Can you work these out from the model? Positions are in its coordinate system, mm. A direction names the side the tool comes from. Round coordinates to 2 decimals unless told otherwise and drop trailing zeros. Write each loop counter-clockwise with the first axis right and the second up, starting at its lowest first coordinate (ties: lowest second). Pieces come first, ordered by that corner, then holes. Notation, with made-up numbers: M -2,3 L 8,3 A4 ccw 8,10 Z; hole C 51,-4.75 d2. An arc over 180 degrees is marked long. Use one line per item in the form item = value. Start each with the question number.
```python
from build123d import *

# Parameters (mm, degrees)
BOX044_W         = 24
BOX044_H         = 42
BOX044_DEPTH     = 13
SKETCH022_R      = 5
SKETCH022_R_2    = 4.5
SKETCH022_R_3    = 1.25
EXTRUDE022_DEPTH = 3
BOX039_W         = 3
BOX039_H         = 2
BOX039_DEPTH     = 2


with BuildPart() as cube005:
    # Box044 → Box044 (new body)
    with BuildSketch(Plane(origin=(-12, -2, 12), x_dir=(1, 0, 0), z_dir=(0, 0, 1))):
        with Locations((12, 21)):
            Rectangle(BOX044_W, BOX044_H)
    extrude(amount=BOX044_DEPTH)


with BuildPart() as back_cover:
    # Sketch022 → Extrude022 (new body)
    with BuildSketch(Plane.XZ):
        with BuildLine():
            ThreePointArc((10, 11), (0, 22.517745), (-10, 11))
            ThreePointArc((-10, 11), (-15.587711, 0.627088), (-10.5, -10))
            Line((-10.5, -10), (-10.5, -13))
            Line((-10.5, -13), (-15, -13))
            Line((-15, -13), (-15, -20))
            Line((-15, -20), (15, -20))
            Line((15, -13), (15, -20))
            Line((10.5, -13), (15, -13))
            Line((10.5, -10), (10.5, -13))
            ThreePointArc((10.5, -10), (15.587711, 0.627088), (10, 11))
        make_face()
        Circle(SKETCH022_R, mode=Mode.SUBTRACT)
        with Locations((0, 12.417745)):
            Circle(SKETCH022_R_2, mode=Mode.SUBTRACT)
        with Locations((-10.8747, -16.5)):
            Circle(SKETCH022_R_3, mode=Mode.SUBTRACT)
        with Locations((10.8747, -16.5)):
            Circle(SKETCH022_R_3, mode=Mode.SUBTRACT)
    extrude(amount=-EXTRUDE022_DEPTH)


with BuildPart() as back_cover_1:
    # Extrude022 placement: moved
    add(back_cover.part.moved(Location((0, 31, 0))))


with BuildPart() as cover:
    # Box039 → Box039 (new body)
    with BuildSketch(Plane(origin=(-1.5, 29, 19.5), x_dir=(1, 0, 0), z_dir=(0, 0, 1))):
        with Locations((1.5, 1)):
            Rectangle(BOX039_W, BOX039_H)
    extrude(amount=BOX039_DEPTH)

    # Fusion025: union Back_cover
    add(back_cover_1.part)

    # Cut032: cut Cube005
    add(cube005.part, mode=Mode.SUBTRACT)


solid = cover.part
```
1. If we section it at B-B (y = 32.1): List the corners of the cut face in (x, z) for me.
2. If we section it at C-C (z = -16.5): List the corners of the cut face in (x, y) for me, and give its area (3 significant figures).
3. Will these pins go through, and if not, where does the flat tip stop? pin 1 (0.9 mm diameter, centred on y = 32, z = -11, fed in from -X); pin 2 (0.9 mm diameter, centred on y = 32.5, z = -12, fed in from +X); pin 3 (1.5 mm diameter, centred on x = 10.87, z = -16.5, fed in from +Y); pin 4 (0.9 mm diameter, centred on y = 32.5, z = -16.5, fed in from +X).
4. If we section it at D-D (z = 9.5): List the corners of the cut face in (x, y) for me.
5. If we section it at A-A (x = 0): List the corners of the cut face in (y, z) for me, and give its area (3 significant figures).
6. If we mould it in two halves opening along Z, with no side actions, what happens to faces 5 (the face through (-7, 33, 12)), 6 (the face through (-15, 32, -16)), 7 (the face through (10.057, 32.479, 11.492))? For each: pulls with the +Z half, pulls with the -Z half, needs draft (parallel to the pull), parting line crosses it, or undercut.
7. Please list where these lines run through material, in increasing order: line 1 along Z through (x, y) = (-11, 32.7); line 2 along Z through (x, y) = (2, 33.2); line 3 along Z through (x, y) = (12, 32.15).
8. Which directions (+Z, -Z, +X, -X, +Y, -Y) give clear straight access to the entire face, cutting with the end or side of a thin tool? Please do faces 1 (the face through (-10.06, 32.48, 11.51)), 2 (the face through (15, 32, -16)), 3 (the face through (10.5, 32, -11)), 4 (the face through (7, 33, 12)).
Model answer:
q1.outline = M -15,-20 L 15,-20 L 15,-13 L 10.5,-13 L 10.5,-10 A13 ccw 10,11 A10.1 ccw 10.09,12 L 4.48,12 A4.5 cw -4.48,12 L -10.09,12 A10.1 ccw -10,11 A13 ccw -10.5,-10 L -10.5,-13 L -15,-13 Z; hole C -10.87,-16.5 d2.5; hole C 0,0 d10; hole C 10.87,-16.5 d2.5
q2.outline = M -15,31 L -12.12,31 L -12.12,34 L -15,34 Z; M -9.62,31 L 9.62,31 L 9.62,34 L -9.62,34 Z; M 12.12,31 L 15,31 L 15,34 L 12.12,34 Z
q2.area = 75.0 mm2
q3.pin_1 = -10.5
q3.pin_2 = 10.5
q3.pin_3 = through
q3.pin_4 = 15
q4.outline = M -11.79,31 L -3.43,31 L -3.43,34 L -11.79,34 Z; M 3.43,31 L 11.79,31 L 11.79,34 L 3.43,34 Z
q5.outline = M 31,-20 L 34,-20 L 34,-5 L 31,-5 Z; M 31,5 L 34,5 L 34,7.92 L 31,7.92 Z
q5.area = 53.8 mm2
q6.face_5 = pulls with the +Z half
q6.face_6 = needs draft
q6.face_7 = undercut
q7.line_1 = -20 to -17.74, -15.26 to -13, -9.6 to 10.23
q7.line_2 = -20 to -4.58, 4.58 to 8.39
q7.line_3 = -20 to -17.04, -15.96 to -13, -8.65 to 9.29
q8.face_1 = -X, +Y, -Y
q8.face_2 = -Z, +X, +Y, -Y
q8.face_3 = +X, +Y, -Y
q8.face_4 = +Z, +X, -X, +Y, -Y
